Job drawing, mm, ordinate dimensions from the low corner. One solid piece. A direction names the side the tool comes from. Coordinates: 2 decimals unless noted, no trailing zeros. Loops run counter-clockwise (first coordinate to the right, second up) from the corner with the lowest first, then second, coordinate; pieces in that order, holes last. Notation, with made-up numbers: (45, 4.25) - (103, 4.25) arc R24 cw to (103, 32.25) - close; hole circle Ø9 at (50, 64.5). An arc over 180 degrees is marked (long way). One line per question, with ' | ' between items. Start each with the question number.
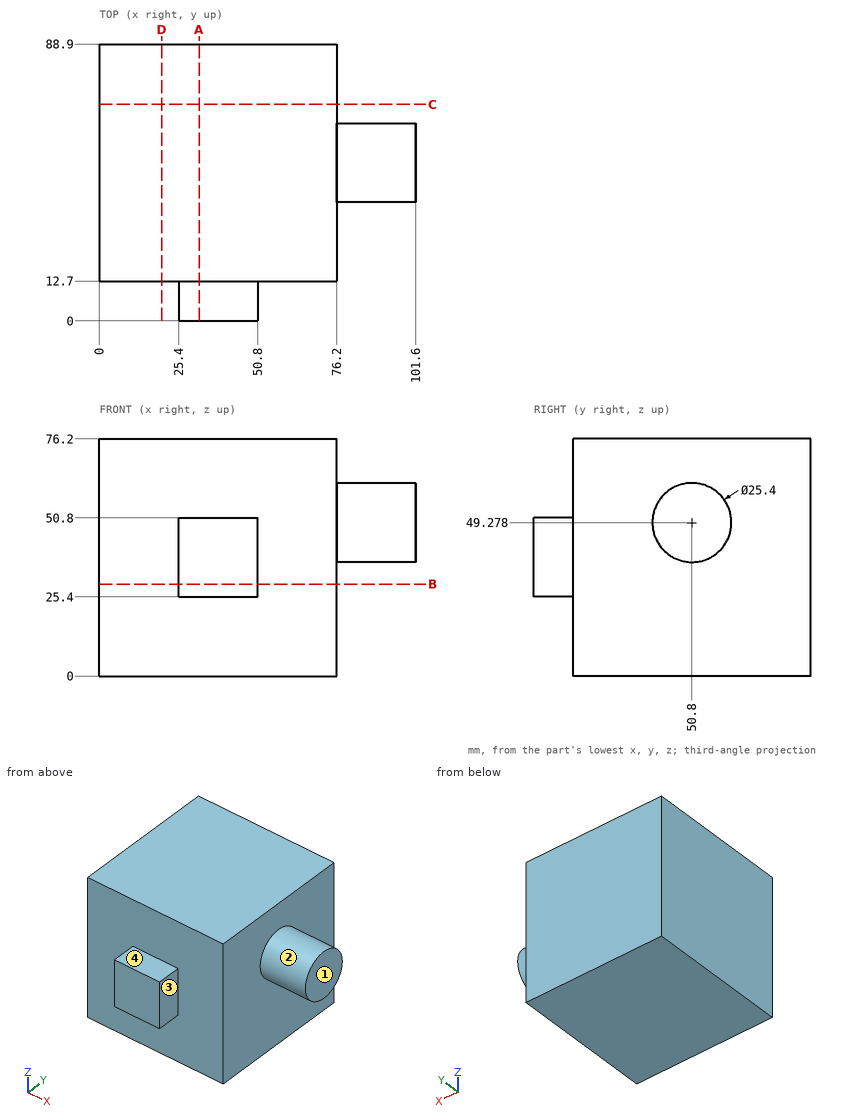
1) Band-saw the part on B-B on z = 29.5. List the corners of the cut face in (x, y).
2) Band-saw the part on D-D on x = 20. List the corners of the cut face in (y, z).
3) Band-saw the part on A-A on x = 32. List the corners of the cut face in (y, z).
4) Band-saw the part on C-C on y = 69.5. List the corners of the cut face in (x, z).
5) Wall check: line 1 along Y through (x, z) = (51.5, 50); line 2 along X through (y, z) = (17.5, 41.5); line 3 along X through (y, z) = (6, 28.5). Give the ranges that are in metal, low to high. Write a range as [from, to].
6) Tool access for the marked faces 1, 2, 3 and 4: list every direction of +Z, -Z, +X, -X, +Y, -Y with a clear straight run to the whole face (end or side of a thin tool).
7) Pin check, flat tips, straight feed: pin 1 Ø4 at (y, z) = (5, 36.5) entering from -X; pin 2 Ø4 at (y, z) = (4.5, 33) entering from +X; pin 3 Ø2 at (y, z) = (29, 37.5) entering from +X. Stop position of each tip, or through.
Values found:
1) outline: (0, 12.7) - (25.4, 12.7) - (25.4, 0) - (50.8, 0) - (50.8, 12.7) - (76.2, 12.7) - (76.2, 88.9) - (0, 88.9) - close
2) outline: (12.7, 0) - (88.9, 0) - (88.9, 76.2) - (12.7, 76.2) - close
3) outline: (0, 25.4) - (12.7, 25.4) - (12.7, 0) - (88.9, 0) - (88.9, 76.2) - (12.7, 76.2) - (12.7, 50.8) - (0, 50.8) - close
4) outline: (0, 0) - (76.2, 0) - (76.2, 76.2) - (0, 76.2) - close
5) line 1: [12.7, 88.9] | line 2: [0, 76.2] | line 3: [25.4, 50.8]
6) face 1: +Z, -Z, +X, +Y, -Y | face 2: +X | face 3: +Z, -Z, +X, -Y | face 4: +Z, +X, -X, -Y
7) pin 1: x = 25.4 | pin 2: x = 50.8 | pin 3: x = 76.2
